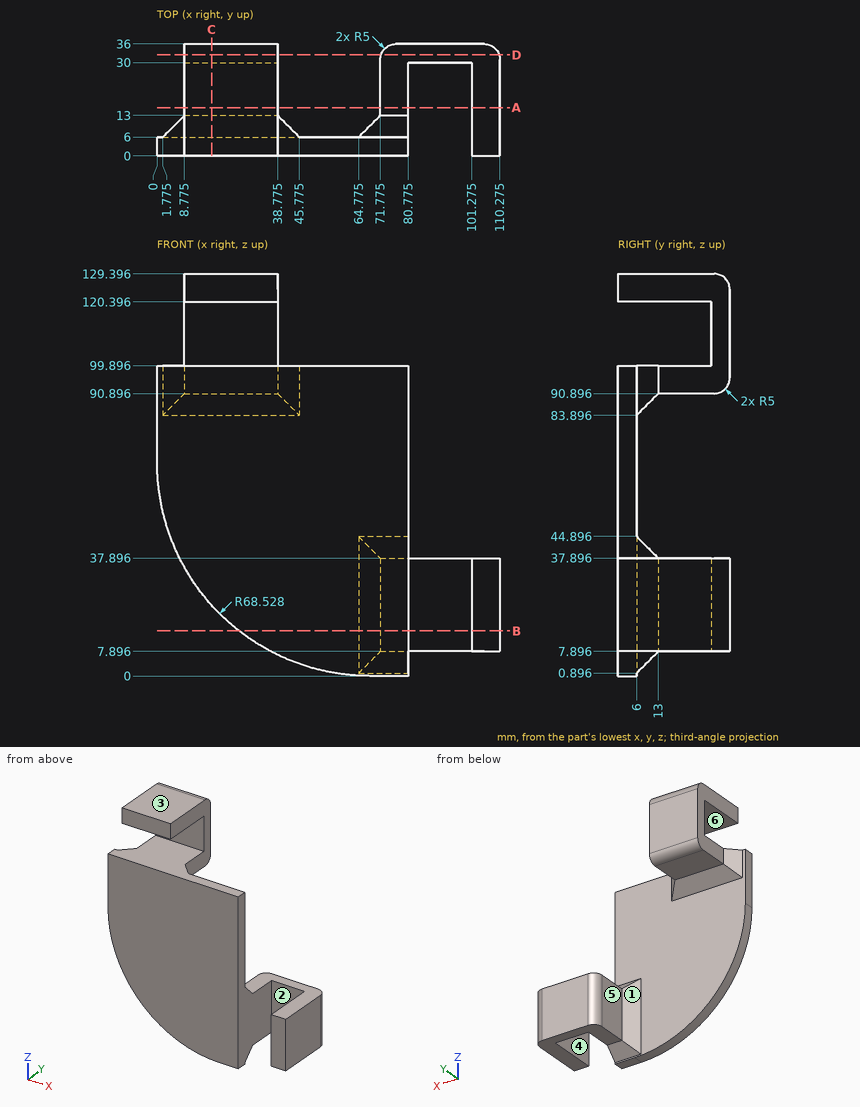
Design review of the part shown in the three views and the two pictorial views. Dimensions are in mm from the part's minimum x, y and z. A direction names the side the tool comes from. Give positions to 0.01 mm unless a question says otherwise; leave off trailing zeros. Write each loop counter-clockwise with the first axis right and the second up, starting at its lowest first coordinate (ties: lowest second). Pieces come first, ordered by that corner, then holes. Notation, with made-up numbers: (20, 10) - (41, 10) arc R29 cw to (41, 49) - close; hole circle Ø5 at (-25.5, -2). An arc over 180 degrees is marked (long way). Return JSON: item names as keys, results as strings. Group by question number.
(1) Mouldability with a two-part tool opening along X and no side actions: class the marked faces 1, 2 and 3 as +X half, -X half, draft (parallel to the pull), parting line (faces both ways), or undercut.
(2) Insertion check: pin 1 (10.5 mm diameter, centred on x = 16.5, z = 113, fed in from -Y); pin 2 (9 mm diameter, centred on x = 21, y = 23, fed in from -Z); pin 3 (18 mm diameter, centred on x = 93.5, y = 19.5, fed in from +Z); pin 4 (16.5 mm diameter, centred on x = 86.5, z = 20.5, fed in from -Y). Each pin has a flat end and moves straight along its axis. Give the tip position at first contact, or say it passes through.
(3) We need section A-A, the plane y = 15.5. Give the boundary of the cut face in (x, z) (1 decimal).
(4) We need section B-B, the plane z = 14.5. Give the boundary of the cut face in (x, y) (1 decimal), then the cut area to 3 significant figures.
(5) To check wall thickness, follow probe 1 along Z at (x, y) = (15, 28.5); probe 2 along Y at (x, z) = (35, 105.5); probe 3 along Z at (x, y) = (15.5, 10) (1 decimal). State the ranges of each line that lie inside material, in increasing order.
(6) We need section C-C, the plane x = 17.5. Give the boundary of the cut face in (y, z).
(7) We need section D-D, the plane y = 32.5. Give the boundary of the cut face in (x, z) (1 decimal), then the cut area to 3 significant figures.
(8) Machinability: for the marked faces 4, 5 and 6, which of the approach directions +Z, -Z, +X, -X, +Y, -Y give a long, thin tool a straight path to every point of the face, cutting with its end or side? Answer none if there is none.
Reported:
{
 "1": {"face 1": "-X half", "face 2": "undercut", "face 3": "draft"},
 "2": {"pin 1": "stops at y = 30", "pin 2": "stops at z = 90.9", "pin 3": "stops at z = 37.9", "pin 4": "stops at y = 0"},
 "3": {"outline": "(8.8, 90.9) - (38.8, 90.9) - (38.8, 99.9) - (8.8, 99.9) - close; (8.8, 120.4) - (38.8, 120.4) - (38.8, 129.4) - (8.8, 129.4) - close; (71.8, 7.9) - (80.8, 7.9) - (80.8, 37.9) - (71.8, 37.9) - close; (101.3, 7.9) - (110.3, 7.9) - (110.3, 37.9) - (101.3, 37.9) - close"},
 "4": {"outline": "(26.4, 0) - (80.8, 0) - (80.8, 30) - (101.3, 30) - (101.3, 0) - (110.3, 0) - (110.3, 31) arc R5 ccw to (105.3, 36) - (76.8, 36) arc R5 ccw to (71.8, 31) - (71.8, 13) - (64.8, 6) - (26.4, 6) - close", "area": "1,060 mm2"},
 "5": {"probe 1": "z = 90.9 to 99.9, 120.4 to 129.4", "probe 2": "y = 30 to 36", "probe 3": "z = 87.9 to 99.9, 120.4 to 129.4"},
 "6": {"outline": "(0, 22.79) - (6, 22.79) - (6, 83.9) - (13, 90.9) - (31, 90.9) arc R5 ccw to (36, 95.9) - (36, 124.4) arc R5 ccw to (31, 129.4) - (0, 129.4) - (0, 120.4) - (30, 120.4) - (30, 99.9) - (0, 99.9) - close"},
 "7": {"outline": "(8.8, 91.1) - (38.8, 91.1) - (38.8, 129.2) - (8.8, 129.2) - close; (72, 7.9) - (110, 7.9) - (110, 37.9) - (72, 37.9) - close", "area": "2,280 mm2"},
 "8": {"face 4": "+Z, -Z, -Y", "face 5": "+Z, -Z, -X, +Y", "face 6": "+X, -X, -Y"}
}
